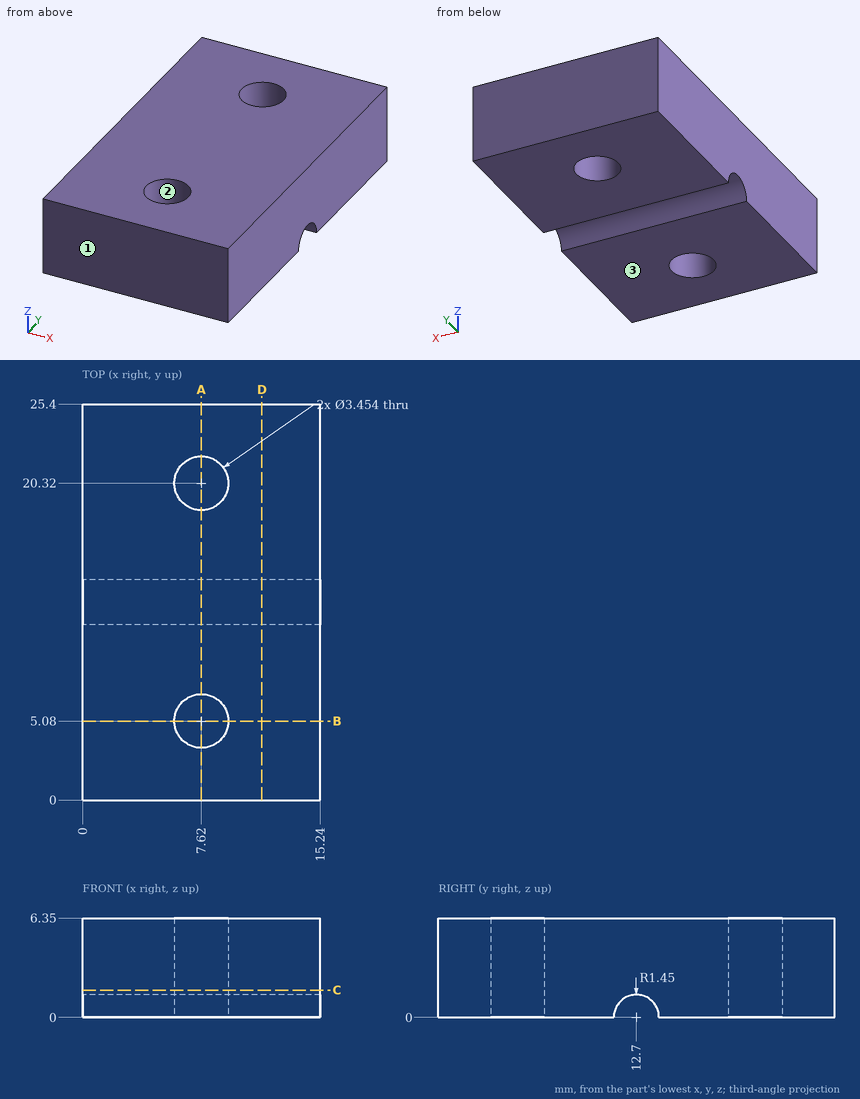
Part print with two shaded views. Sizes in mm from the minimum x, y, z corner. Coordinates: 2 decimals unless noted, no trailing zeros. Order: outer loops, then holes, each group sorted by start corner. A loop starts at its lowest first (then second) coordinate and runs counter-clockwise, first axis right, second up. Notation, with made-up numbers: (9, 29) - (27, 29) arc R21 ccw to (27, 63) - close; hole circle Ø4 at (-36, -29). An arc over 180 degrees is marked (long way). Answer in a Markdown table with one row per item.
1. Slice it at B-B, the plane y = 5.08. List the corners of the cut face in (x, z).
Answer:
| item | result |
|---|---|
| outline | (0, 0) - (5.89, 0) - (5.89, 6.35) - (0, 6.35) - close; (9.35, 0) - (15.24, 0) - (15.24, 6.35) - (9.35, 6.35) - close |
2. Drill centre lines: L1, parallel to Y at x = 7.5, z = 3; L2, parallel to Y at x = 5.5, z = 1; L3, parallel to X at y = 21, z = 2.5. Where is each one in solid material? Low to high. Write a range as from..to.
Answer:
| item | result |
|---|---|
| L1 | 0..3.36, 6.8..18.6, 22.04..25.4 |
| L2 | 0..11.65, 13.75..25.4 |
| L3 | 0..6.03, 9.21..15.24 |
3. Slice it at D-D, the plane x = 11.5. List the corners of the cut face in (y, z).
Answer:
| item | result |
|---|---|
| outline | (0, 0) - (11.25, 0) arc R1.45 cw to (14.15, 0) - (25.4, 0) - (25.4, 6.35) - (0, 6.35) - close |
4. Slice it at A-A, the plane x = 7.62. List the corners of the cut face in (y, z).
Answer:
| item | result |
|---|---|
| outline | (0, 0) - (3.35, 0) - (3.35, 6.35) - (0, 6.35) - close; (6.81, 0) - (11.25, 0) arc R1.45 cw to (14.15, 0) - (18.59, 0) - (18.59, 6.35) - (6.81, 6.35) - close; (22.05, 0) - (25.4, 0) - (25.4, 6.35) - (22.05, 6.35) - close |
5. Pull direction Y, two halves, no side cores. Call the marked faces 1, 2 and 3: +Y half, -Y half, draft (parallel to the pull), parting line (faces both ways), or undercut.
Answer:
| item | result |
|---|---|
| face 1 | -Y half |
| face 2 | undercut |
| face 3 | draft |
6. Slice it at C-C, the plane z = 1.75. List the corners of the cut face in (x, y) (1 decimal).
Answer:
| item | result |
|---|---|
| outline | (0, 0) - (15.2, 0) - (15.2, 25.4) - (0, 25.4) - close; hole circle Ø3.5 at (7.6, 5.1); hole circle Ø3.5 at (7.6, 20.3) |
